Build history of the part. All positions in model axes, mm. Face numbers are marked on the shaded views. A direction names the side the tool comes from. Coordinates: 2 decimals unless noted, no trailing zeros. Order: outer loops, then holes, each group sorted by start corner. A loop starts at its lowest first (then second) coordinate and runs counter-clockwise, first axis right, second up. Notation, with made-up numbers: (52, -20) - (106, -20) arc R23 cw to (106, 6) - close; hole circle Ø2 at (43, 63.5). An arc over 180 degrees is marked (long way). Write each question's results on one line, items separated by ' | '. Start each with the question number.
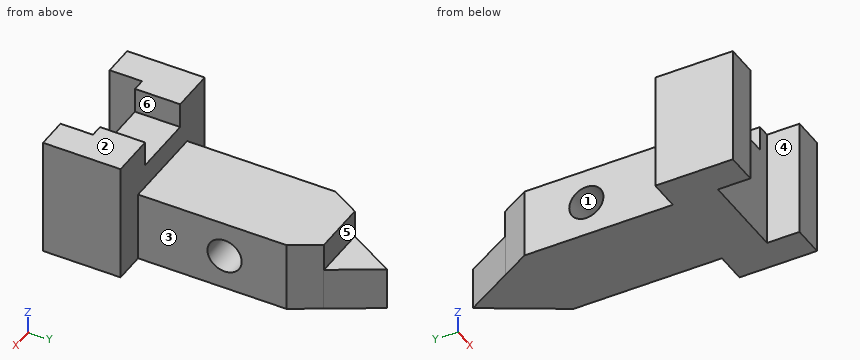
from build123d import *

# Parameters (mm, degrees)
BOSS_EXTRUDE1_DEPTH      = 22.4
SKETCH2_R                = 10.908211602
CUT_EXTRUDE1_DEPTH       = 156.383396796
SKETCH3_W                = 70.975037356
SKETCH3_H                = 39.358884352
CUT_EXTRUDE2_DEPTH       = 17.6
BOSS_EXTRUDE3_DEPTH      = 53.6
BOSS_EXTRUDE3_DEPTH_BACK = 22.4
SKETCH7_W                = 40
SKETCH7_H                = 93.823615884
CUT_EXTRUDE4_DEPTH       = 16


with BuildPart() as part:
    # Sketch1 → Boss-Extrude1 (new, symmetric)
    with BuildSketch(Plane.XY):
        Polygon((-17.666918237, 112.6), (-28, 94.702577388), (-28, 0), (0, 0), (28, 0), (28, 94.702577388), (17.666918237, 112.6), (0, 143.2), align=None)
    extrude(amount=BOSS_EXTRUDE1_DEPTH, both=True)

    # Sketch2 → Cut-Extrude1 (cut, through all)
    with BuildSketch(Plane(origin=(28, 0, 0), x_dir=(0, 0, -1), z_dir=(1, 0, 0))):
        with Locations(Location((0, 55.2, 0), (0, 0, 90))):
            Circle(SKETCH2_R)
    extrude(amount=-CUT_EXTRUDE1_DEPTH, mode=Mode.SUBTRACT)

    # Sketch3 → Cut-Extrude2 (cut)
    with BuildSketch(Plane.XY.offset(22.4)):
        with Locations((-1.700797659, 132.479442176)):
            Rectangle(SKETCH3_W, SKETCH3_H)
    extrude(amount=-CUT_EXTRUDE2_DEPTH, mode=Mode.SUBTRACT)

    # Sketch4 → Boss-Extrude3 (add, two sides: drawn at the far end of the back side and taken through both)
    with BuildSketch(Plane.XY.offset(-BOSS_EXTRUDE3_DEPTH_BACK)):
        Polygon((0, 0), (-28, 0), (-48, 0), (-48, -49.489884121), (-28, -49.489884121), (-28, -28.8), (28, -28.8), (28, -49.489884121), (48, -49.489884121), (48, 0), (28, 0), align=None)
    extrude(amount=BOSS_EXTRUDE3_DEPTH + BOSS_EXTRUDE3_DEPTH_BACK)

    # Sketch7 → Cut-Extrude4 (cut)
    with BuildSketch(Plane.XY.offset(53.6)):
        with Locations((0, -14.4)):
            Rectangle(SKETCH7_W, SKETCH7_H)
    extrude(amount=-CUT_EXTRUDE4_DEPTH, mode=Mode.SUBTRACT)


solid = part.part
Item 1: Probe probe 1 along Z at (x, y) = (14.5, 55.2); probe 2 along X at (y, z) = (-3, 49); probe 3 along X at (y, z) = (86.5, 5.5). List the from-to ranges inside material, lowest first.
Item 2: Slice it at B-B (y = 55.2). Write the cut outline in (x, z), then the cut area to 3 significant figures.
Item 3: Flat gauge pins, fed straight in: P1, Ø9, axis at x = 8, z = 11.5, coming from the +Y side; P2, Ø6, axis at y = 104, z = 15.5, coming from the -X side; P3, Ø5, axis at y = 119, z = 8, coming from the -X side; P4, Ø1.5, axis at x = -14.5, y = 51, coming from the +Z side. Where does each tip first touch, or does it go through?
Item 4: Slice it at A-A (z = 47). Write the cut outline in (x, y).
Item 5: Slice it at C-C (x = 4.5). Write the cut outline in (y, z).
Item 6: Pull direction Z, two halves, no side cores. Call the marked faces 1, 2 and 3: released by +Z, released by -Z, zero draft, split by the parting line, or undercut.
Item 7: Which spindle directions (+Z, -Z, +X, -X, +Y, -Y) get a long thin tool onto all of the face, cutting with end or side? Do the marked faces 4, 5 and 6. Say none if no direction does.
Item 8: Slice it at D-D (z = 0). Write the cut outline in (x, y), then the cut area to 3 significant figures.
Resolved:
1) probe 1: -22.4 to -10.91, 10.91 to 22.4 | probe 2: -48 to -20, 20 to 48 | probe 3: -28 to 28
2) outline: (-28, -22.4) - (28, -22.4) - (28, -10.91) - (-28, -10.91) - close; (-28, 10.91) - (28, 10.91) - (28, 22.4) - (-28, 22.4) - close | area: 1,290 mm^2
3) P1: y = 112.8 | P2: x = -24.36 | P3: through | P4: z = 22.4
4) outline: (-48, -49.49) - (-28, -49.49) - (-28, -28.8) - (-20, -28.8) - (-20, 0) - (-48, 0) - close; (20, -28.8) - (28, -28.8) - (28, -49.49) - (48, -49.49) - (48, 0) - (20, 0) - close
5) outline: (-28.8, -22.4) - (135.41, -22.4) - (135.41, 4.8) - (112.8, 4.8) - (112.8, 22.4) - (0, 22.4) - (0, 37.6) - (-28.8, 37.6) - close; hole circle Ø21.82 at (55.2, 0)
6) face 1: undercut | face 2: released by +Z | face 3: zero draft
7) face 4: +Z, -Z, -Y | face 5: +Z, +X, -X, +Y | face 6: +Z, +Y, -Y
8) outline: (-48, -49.49) - (-28, -49.49) - (-28, -28.8) - (28, -28.8) - (28, -49.49) - (48, -49.49) - (48, 0) - (28, 0) - (28, 44.29) - (-28, 44.29) - (-28, 0) - (-48, 0) - close; (-28, 66.11) - (28, 66.11) - (28, 94.7) - (0, 143.2) - (-28, 94.7) - close | area: 9,030 mm^2
